Work out the finished part from the listing and answer in its coordinate system (mm). A direction names the side the tool comes from. Round coordinates to 2 decimals unless told otherwise and drop trailing zeros. Write each loop counter-clockwise with the first axis right and the second up, starting at its lowest first coordinate (ties: lowest second). Pieces come first, ordered by that corner, then holes.
1. Find section C-C (y = 9.75). Write down the section's boundary in (x, z), and give its area (3 significant figures).
2. Determine the mould class of faces 1 (the face through (0.1, 2.5, -11.3)), 2 (the face through (-12.727, 25.398, 12.465)), 3 (the face through (-21.73, 2.46, 4.93)), 4 (the face through (2, 1, 5)) for opening direction X: pulls with the +X half, pulls with the -X half, needs draft (parallel to the pull), parting line crosses it, or undercut.
3. Find section A-A (x = 0). Write down the section's boundary in (y, z), and give its area (3 significant figures).
4. Straight lines are drawn through the part: probe 1 along Y at (x, z) = (-12.95, 13.95); probe 2 along Z at (x, y) = (1.5, 9.5); probe 3 along X at (y, z) = (1.5, 10.5). For each, find the intervals that lie inside material, in ascending order.
5. Flat-ended cylindrical pins translate along their axes: pin 1 Ø2.5 at (y, z) = (1.5, -4.5) entering from +X; pin 2 Ø1.5 at (y, z) = (1.5, 5.5) entering from -X; pin 3 Ø2.5 at (x, z) = (-1, 13.5) entering from +Y; pin 4 Ø2 at (x, z) = (0, 0) entering from -Y. Find the tip coordinate at first contact, or state that the pin passes through.
6. Find section D-D (y = 22.25). Write down the section's boundary in (x, z), and give its area (3 significant figures).
7. Find section B-B (z = 13). Write down the section's boundary in (x, y), and give its area (3 significant figures).
8. A tool of negligible diameter and unlimited length cuts with its end or side. For faces 5 (the face through (-1, 5, 2)), 6 (the face through (-2, 1, 5)), 7 (the face through (4, 2, -6)), from which of +Z, -Z, +X, -X, +Y, -Y can it reach the whole face along a straight path? Write none if from no direction.
```python
from build123d import *
from build123d.topology import SkipClean

# Parameters (mm, degrees)
BOSS_EXTRUDE1_DEPTH = 3
SKETCH3_R           = 1.2
BOSS_EXTRUDE2_DEPTH = 2
SKETCH6_R           = 8.15
BOSS_EXTRUDE4_DEPTH = 5
BOSS_EXTRUDE5_START = -5
BOSS_EXTRUDE5_DEPTH = 5


with BuildPart() as part:
    # Sketch2 → Boss-Extrude1 (new body)
    with BuildSketch(Plane(origin=(0, 0, 0), x_dir=(1, 0, 0), z_dir=(0, 1, 0))):
        with BuildLine():
            Line((4, -7.3), (4, -4.797924238))
            Line((4, -4.797924238), (14.092577275, -3.998928538))
            ThreePointArc((14.092577275, -3.998928538), (18, 0), (14.092577275, 3.998928538))
            Line((14.092577275, 3.998928538), (4, 4.797924238))
            Line((4, 4.797924238), (4, 7.3))
            ThreePointArc((4, 7.3), (0, 11.3), (-4, 7.3))
            Line((-4, 7.3), (-4, 5.302488085))
            Line((-4, 5.302488085), (-16.521647449, 3.998149809))
            ThreePointArc((-16.521647449, 3.998149809), (-20.4, 0), (-16.521647449, -3.998149809))
            Line((-16.521647449, -3.998149809), (-4, -5.302488085))
            Line((-4, -5.302488085), (-4, -7.3))
            ThreePointArc((-4, -7.3), (0, -11.3), (4, -7.3))
        make_face()
        with BuildLine():
            ThreePointArc((-16.4, -2), (-18.4, 0), (-16.4, 2))
            Line((-16.4, 2), (-2, 3.5))
            Line((-2, 3.5), (-2, 7.3))
            ThreePointArc((-2, 7.3), (0, 9.3), (2, 7.3))
            Line((2, 7.3), (2, 2.95))
            Line((2, 2.95), (14, 2))
            ThreePointArc((14, 2), (16, 0), (14, -2))
            Line((14, -2), (2, -2.95))
            Line((2, -2.95), (2, -7.3))
            ThreePointArc((2, -7.3), (0, -9.3), (-2, -7.3))
            Line((-2, -7.3), (-2, -3.5))
            Line((-2, -3.5), (-16.4, -2))
        make_face(mode=Mode.SUBTRACT)
    extrude(amount=BOSS_EXTRUDE1_DEPTH)

    # Sketch3 → Boss-Extrude2 (add)
    with BuildSketch(Plane(origin=(0, 3, 0), x_dir=(1, 0, 0), z_dir=(0, 1, 0))):
        with BuildLine():
            Line((-4, 5.302488085), (-16.521647449, 3.998149809))
            ThreePointArc((-16.521647449, 3.998149809), (-20.4, 0), (-16.521647449, -3.998149809))
            Line((-16.521647449, -3.998149809), (-4, -5.302488085))
            Line((-4, -5.302488085), (-4, -7.3))
            ThreePointArc((-4, -7.3), (0, -11.3), (4, -7.3))
            Line((4, -7.3), (4, -4.797924238))
            Line((4, -4.797924238), (14.092577275, -3.998928538))
            ThreePointArc((14.092577275, -3.998928538), (18, 0), (14.092577275, 3.998928538))
            Line((14.092577275, 3.998928538), (4, 4.797924238))
            Line((4, 4.797924238), (4, 7.3))
            ThreePointArc((4, 7.3), (0, 11.3), (-4, 7.3))
            Line((-4, 7.3), (-4, 5.302488085))
        make_face()
        with Locations(Location((0, 0, 0), (0, 0, 270))):
            Circle(SKETCH3_R, mode=Mode.SUBTRACT)
    extrude(amount=BOSS_EXTRUDE2_DEPTH)

    # Sketch6 → Boss-Extrude4 (add)
    with BuildSketch(Plane.XY.offset(10)):
        with BuildLine():
            Line((21.1, 5), (21.1, 9.200206615))
            ThreePointArc((21.1, 9.200206615), (16.135906464, 24.887037927), (2.8, 15.25))
            Line((2.8, 15.25), (-2.8, 15.25))
            ThreePointArc((-2.8, 15.25), (-12.95, 25.4), (-23.1, 15.25))
            Line((-23.1, 15.25), (-23.1, 5))
            Line((-23.1, 5), (21.1, 5))
        make_face()
        with Locations((-12.95, 15.25)):
            Circle(SKETCH6_R, mode=Mode.SUBTRACT)
        with Locations((12.95, 15.25)):
            Circle(SKETCH6_R, mode=Mode.SUBTRACT)
    extrude(amount=BOSS_EXTRUDE4_DEPTH)

    # Sketch8 → Boss-Extrude5 (add)
    with SkipClean():  # the faces are left unmerged after this step: merging them gives an invalid solid
        with BuildSketch(Plane(origin=(0, 5, 0), x_dir=(1, 0, 0), z_dir=(0, 1, 0)).offset(BOSS_EXTRUDE5_START)):
            with BuildLine():
                ThreePointArc((-16.521647449, -3.998149809), (-19.271113878, -2.785086193), (-20.4, 0))
                Line((-20.4, 0), (-23.1, -10))
                Line((-23.1, -10), (-2.951270913, -10))
                ThreePointArc((-2.951270913, -10), (-3.728611246, -8.748260396), (-4, -7.3))
                Line((-4, -7.3), (-4, -5.302488085))
                Line((-4, -5.302488085), (-16.521647449, -3.998149809))
            make_face()
            with BuildLine():
                ThreePointArc((4, -7.3), (3.728611246, -8.748260396), (2.951270913, -10))
                Line((2.951270913, -10), (21.1, -10))
                Line((21.1, -10), (18, 0))
                ThreePointArc((18, 0), (16.860970911, -2.795504507), (14.092577275, -3.998928538))
                Line((14.092577275, -3.998928538), (4, -4.797924238))
                Line((4, -4.797924238), (4, -7.3))
            make_face()
            with BuildLine():
                ThreePointArc((-2.951270913, -10), (0, -11.3), (2.951270913, -10))
                Line((2.951270913, -10), (21.1, -10))
                Line((21.1, -10), (21.1, -15))
                Line((21.1, -15), (-23.1, -15))
                Line((-23.1, -15), (-23.1, -10))
                Line((-23.1, -10), (-2.951270913, -10))
            make_face()
        extrude(amount=BOSS_EXTRUDE5_DEPTH)


solid = part.part
```
Worked answers:
1. outline: (-23.1, 10) - (-18.96, 10) - (-18.96, 15) - (-23.1, 15) - close; (-6.94, 10) - (6.94, 10) - (6.94, 15) - (-6.94, 15) - close; (18.96, 10) - (21.48, 10) - (21.48, 15) - (18.96, 15) - close
1. area: 103 mm2
2. face 1: parting line crosses it
2. face 2: undercut
2. face 3: pulls with the -X half
2. face 4: undercut
3. outline: (0, -11.3) - (5, -11.3) - (5, -1.2) - (3, -1.2) - (3, -9.3) - (0, -9.3) - close; (0, 9.3) - (3, 9.3) - (3, 1.2) - (5, 1.2) - (5, 10) - (15.25, 10) - (15.25, 15) - (0, 15) - close
3. area: 122 mm2
4. probe 1: y = 0 to 7.1, 23.4 to 25.4
4. probe 2: z = 10 to 15
4. probe 3: x = -23.1 to 21.1
5. pin 1: stops at x = 16.33
5. pin 2: stops at x = -22.09
5. pin 3: stops at y = 15.25
5. pin 4: passes through
6. outline: (-20.3, 10) - (-17.12, 10) - (-17.12, 15) - (-20.3, 15) - close; (-8.78, 10) - (-5.6, 10) - (-5.6, 15) - (-8.78, 15) - close; (5.6, 10) - (8.78, 10) - (8.78, 15) - (5.6, 15) - close; (17.12, 10) - (20.3, 10) - (20.3, 15) - (17.12, 15) - close
6. area: 63.5 mm2
7. outline: (-23.1, 0) - (21.1, 0) - (21.1, 9.2) arc R10.15 ccw (long way) to (2.8, 15.25) - (-2.8, 15.25) arc R10.15 ccw to (-23.1, 15.25) - close; hole circle Ø16.3 at (-12.95, 15.25); hole circle Ø16.3 at (12.95, 15.25)
7. area: 589 mm2
8. face 5: -Z, +X, -X, +Y
8. face 6: -Y
8. face 7: -Z, +X, +Y, -Y
